Could you check a few things on this model? Use its own coordinates, in mm. A direction names the side the tool comes from. Coordinates: 2 decimals unless noted, no trailing zeros. Order: outer loops, then holes, each group sorted by start corner. A loop starts at its lowest first (then second) coordinate and runs counter-clockwise, first axis right, second up. Notation, with made-up numbers: (-23.5, -33.75) - (-19.5, -33.75) arc R13 ccw to (-19.5, -20.75) - close; hole circle Ø9 at (8, 3.5). An arc over 180 degrees is marked (long way). Answer as a JSON object with one key per item and string values. Group by question number.
(1) Imagine slicing it at C-C, the plane z = 0.9. Write out the boundary of the cut face in (x, y), and give its area (3 significant figures).
(2) Which directions (+Z, -Z, +X, -X, +Y, -Y) give clear straight access to the entire face, cutting with the end or side of a thin tool? Please do faces 5 (the cylindrical face through (28.532, -7.494, 2.465)), 6 (the flat face through (-30, -5, 2)), 7 (the flat face through (-2.5, -36, 2)).
(3) Imagine slicing it at D-D, the plane x = -4.5. Write out the boundary of the cut face in (y, z).
(4) Will these pins go through, and if not, where does the flat tip stop? P1, Ø3, axis at x = 19.5, y = -18, coming from the -Z side; P2, Ø3, axis at y = -35.5, z = 2, coming from the -X side; P3, Ø2, axis at x = 14.5, z = 1.5, coming from the -Y side; P4, Ø1.5, axis at y = -13.5, z = 1.5, coming from the +X side.
(5) Imagine slicing it at A-A, the plane y = -20. Write out the boundary of the cut face in (x, z).
(6) Please list where these lines run through material, in increasing order: probe 1 along X at (y, z) = (-15, 1.25); probe 2 along X at (y, z) = (-22.5, 3.6); probe 3 along X at (y, z) = (-33.5, 3.55).
(7) Imagine slicing it at B-B, the plane y = -11. Write out the boundary of the cut face in (x, z).
(8) We'd pull the mould along X, two halves only. Please class faces 1 (the flat face through (-4.8, -29.5, 5)), 2 (the cylindrical face through (-28.514, -7.564, 2.465)), 3 (the cylindrical face through (-29.423, -12.58, 2.465)), 4 (the flat face through (2.5, -35, 2)): pulls with the +X half, pulls with the -X half, needs draft (parallel to the pull), parting line crosses it, or undercut.
Autodesk Inventor part; units mm, degrees
ref_plane "YZ Plane" through (0, 0, 0) normal (1, 0, 0) x (0, 1, 0)
ref_plane "XZ Plane" through (0, 0, 0) normal (0, 1, 0) x (-1, 0, 0)
ref_plane "XY Plane" through (0, 0, 0) normal (0, 0, 1) x (1, 0, 0)
sketch "Sketch1" plane through (0, 0, 0) normal (0, 0, 1) x (1, 0, 0)
  arc A0 (-25.4018, -15) -> (25.4018, -15) centre (0, 0) ccw
  line L0 (2.5, -32) -> (2.5, -39)
  line L1 (2.5, -39) -> (-2.5, -39)
  line L2 (-2.5, -39) -> (-2.5, -32)
  line L3 (-2.5, -32) -> (-2.5, -31.9022)
  line L4 (2.5, -32) -> (2.5, -31.9022)
  arc A1 (-28.2666, -15) -> (-2.5, -31.9022) centre (0, 0) ccw
  arc A2 (2.5, -31.9022) -> (28.2666, -15) centre (0, 0) ccw
  arc A3 (-27.7534, -10) -> (27.7534, -10) centre (0, 0) ccw
  arc A4 (-30.3974, -10) -> (-2.5, -31.9022) centre (0, 0) ccw
  arc A5 (2.5, -31.9022) -> (30.3974, -10) centre (0, 0) ccw
  circle A6 centre (0, 0) radius 29.5
  arc A7 (2.5, -31.9022) -> (-2.5, -31.9022) centre (0, 0) ccw
  line L5 (-29.0732, -5) -> (-31.607, -5)
  line L6 (29.0732, -5) -> (31.607, -5)
  point P0 (25.4018, -15)
  point P1 (-28.2666, -15)
  point P2 (27.7534, -10)
  point P3 (-30.3974, -10)
  dimension "d43" = 5
  dimension "d64" = 7
extrude "Extrusion7" add sketch "Sketch1" along normal blind 5 contours A0 A3 A6 L6 A7 A5 A2 L4 L0 L1 L2 L3 A1 A4 L5
properties part number "Clip_TestFitV1"
Result set:
{
 "1": {"outline": "(-31.61, -5) arc R32 ccw to (-30.4, -10) arc R32 ccw to (-28.27, -15) arc R32 ccw to (-2.5, -31.9) - (-2.5, -39) - (2.5, -39) - (2.5, -31.9) arc R32 ccw to (28.27, -15) arc R32 ccw to (30.4, -10) arc R32 ccw to (31.61, -5) - (29.07, -5) arc R29.5 cw to (-25.4, -15) arc R29.5 cw to (-27.75, -10) arc R29.5 cw to (-29.07, -5) - close", "area": "252 mm^2"},
 "2": {"face 5": "+Z, -Z, +Y", "face 6": "+Z, -Z, +X, -X, +Y", "face 7": "+Z, -Z, -X, -Y"},
 "3": {"outline": "(-31.68, 0) - (-29.15, 0) - (-29.15, 5) - (-31.68, 5) - close"},
 "4": {"P1": "passes through", "P2": "stops at x = -2.5", "P3": "stops at y = -29.01", "P4": "stops at x = 29.35"},
 "5": {"outline": "(-24.98, 0) - (-21.69, 0) - (-21.69, 5) - (-24.98, 5) - close; (21.69, 0) - (24.98, 0) - (24.98, 5) - (21.69, 5) - close"},
 "6": {"probe 1": "x = -28.27 to -25.4, 25.4 to 28.27", "probe 2": "x = -22.75 to -19.08, 19.08 to 22.75", "probe 3": "x = -2.5 to 2.5"},
 "7": {"outline": "(-30.05, 0) - (-27.37, 0) - (-27.37, 5) - (-30.05, 5) - close; (27.37, 0) - (30.05, 0) - (30.05, 5) - (27.37, 5) - close"},
 "8": {"face 1": "needs draft", "face 2": "undercut", "face 3": "pulls with the -X half", "face 4": "pulls with the +X half"}
}
